Part model, mm, in its own coordinate system. A direction names the side the tool comes from. Give positions to 0.01 mm unless a question says otherwise; leave off trailing zeros. Order: outer loops, then holes, each group sorted by start corner. A loop starts at its lowest first (then second) coordinate and runs counter-clockwise, first axis right, second up. Notation, with made-up numbers: M 28.5,-4.75 L 84.5,-4.75 A20 cw 84.5,-0.75 Z; hole C 84.5,85 d8. An arc over 180 degrees is marked long. Answer as a JSON object with one key per item and string values.
from build123d import *

# Parameters (mm, degrees)
F0_W     = 100
F0_H     = 100
F1_DEPTH = 140
F2_W     = 50
F2_H     = 80
F3_DEPTH = 100
F4_W     = 50
F4_H     = 80
F5_DEPTH = 50


with BuildPart() as f1:
    # F0 (on Top) → F1 (new body)
    with BuildSketch(Plane.XY):
        with Locations((-8.820043, 10.226071)):
            Rectangle(F0_W, F0_H)
    extrude(amount=F1_DEPTH)

    # F2 (on face) → F3 (cut, through all)
    with BuildSketch(Plane.XZ.offset(39.773929)):
        with Locations((16.179957, 100)):
            Rectangle(F2_W, F2_H)
    extrude(amount=-F3_DEPTH, mode=Mode.SUBTRACT)

    # F4 (on face) → F5 (cut, through all)
    with BuildSketch(Plane.YZ.offset(-8.820043)):
        with Locations((35.226071, 100)):
            Rectangle(F4_W, F4_H)
    extrude(amount=-F5_DEPTH, mode=Mode.SUBTRACT)


solid = f1.part
1. Which spindle directions (+Z, -Z, +X, -X, +Y, -Y) get a long thin tool onto all of the face, cutting with end or side? Do faces 1 (the flat face through (-33, 10.226, 99)), 2 (the flat face through (-8.82, -15, 99)), 3 (the flat face through (-21, -39.774, 53)). Say none if no direction does.
Worked answers:
{"face 1": "+Z, +X, -X, +Y", "face 2": "+Z, +X, +Y, -Y", "face 3": "+Z, -Z, +X, -X, -Y"}
2. Cut at B-B on y = -14. Give the cut face in (x, z), plus the area to 3 significant figures.
Worked answers:
{"outline": "M -58.82,0 L 41.18,0 L 41.18,60 L -8.82,60 L -8.82,140 L -58.82,140 Z", "area": "10,000 mm^2"}
3. Cut at D-D on x = 11.5. Give the cut face in (y, z), plus the area to 3 significant figures.
Worked answers:
{"outline": "M -39.77,0 L 60.23,0 L 60.23,60 L -39.77,60 Z", "area": "6,000 mm^2"}
4. Cut at A-A on x = -47. Give the cut face in (y, z), plus the area to 3 significant figures.
Worked answers:
{"outline": "M -39.77,0 L 60.23,0 L 60.23,60 L 10.23,60 L 10.23,140 L -39.77,140 Z", "area": "10,000 mm^2"}
5. Cut at C-C on z = 69.5. Give the cut face in (x, y).
Worked answers:
{"outline": "M -58.82,-39.77 L -8.82,-39.77 L -8.82,10.23 L -58.82,10.23 Z"}
6. Probe line 1 along Z through (x, y) = (-7, -30); line 2 along Y through (x, z) = (-12.5, 74); line 3 along X through (y, z) = (-14.5, 101.5). List the from-to ranges inside material, lowest first.
Worked answers:
{"line 1": "z = 0 to 60", "line 2": "y = -39.77 to 10.23", "line 3": "x = -58.82 to -8.82"}
7. Pin check, flat tip, straight feed: P1, Ø4, axis at x = -46.5, z = 97, coming from the +Y side. Stop position of the tip, or through.
Worked answers:
{"P1": "stops at y = 10.23"}
